For this review, take the finished solid that the model builds, in its own axes (mm). Give positions to 0.01 mm unless a question says otherwise; leave off trailing zeros. Write each loop counter-clockwise with the first axis right and the second up, starting at its lowest first coordinate (ties: lowest second). Pieces come first, ordered by that corner, then holes. Notation, with made-up numbers: (21, 44.25) -> (25, 44.25) arc R25 ccw to (25, 70.25) -> close; hole circle Ø6 at (49.25, -14.75). An arc over 180 degrees is marked (long way). Return JSON: item names as keys, results as strings.
Autodesk Inventor part; units mm, degrees
ref_plane "YZ Plane" through (0, 0, 0) normal (1, 0, 0) x (0, 1, 0)
ref_plane "XZ Plane" through (0, 0, 0) normal (0, 1, 0) x (-1, 0, 0)
ref_plane "XY Plane" through (0, 0, 0) normal (0, 0, 1) x (1, 0, 0)
sketch "Sketch1" plane through (0, 0, 0) normal (0, 1, 0) x (-1, 0, 0)
  circle A0 centre (0, 0) radius 27.5
  dimension "d0" = 55
extrude "Extrusion1" add sketch "Sketch1" along normal blind 6
sketch "Sketch2" plane through (0, 6, 0) normal (0, 1, 0) x (1, 0, 0)
  circle A0 centre (0, 0) radius 27.5
  point P0 (20, 0)
  point P1 (14.1421, 14.1421)
  point P2 (0, 20)
  point P3 (-14.1421, 14.1421)
  point P4 (-20, 0)
  point P5 (-14.1421, -14.1421)
  point P6 (0, -20)
  point P7 (14.1421, -14.1421)
  dimension "d3" = 20
  dimension "d6" = 360
hole "Hole1" at (20, 6, 0) at (14.1421, 6, -14.1421) at (0, 6, -20) at (-14.1421, 6, -14.1421) at (-20, 6, 0) at (-14.1421, 6, 14.1421) at (0, 6, 20) at (14.1421, 6, 14.1421) direction (0, -1, 0) diameter 6.6 depth 8 tip angle 118
properties part number "simple_plate"
1. To check wall thickness, follow probe 1 along X at (y, z) = (2.95, 11.5); probe 2 along Z at (x, y) = (-1, 2.85); probe 3 along X at (y, z) = (2.05, 12.5). State the ranges of each line that lie inside material, in increasing order.
Results found:
{"probe 1": "x = -24.98 to -16.12, -12.16 to 12.16, 16.12 to 24.98", "probe 2": "z = -27.48 to -23.14, -16.86 to 16.86, 23.14 to 27.48", "probe 3": "x = -24.49 to -17, -11.28 to 11.28, 17 to 24.49"}
2. The part is to be moulded in two halves that separate along Z. For faces 1 (the cylindrical face through (-12.9, 3, 17.2)), 2 (the cylindrical face through (1.26, 2.96, 23.05)), 3 (the cylindrical face through (5.961, 2.958, 26.846)), 4 (the flat face through (0, 0, 0)), say which applies: +Z half, -Z half, draft (parallel to the pull), parting line (faces both ways), or undercut.
Results found:
{"face 1": "undercut", "face 2": "undercut", "face 3": "parting line", "face 4": "draft"}
3. Add section C-C, the plane z = 1. State the section outline as (x, y) points.
Results found:
{"outline": "(-27.48, 0) -> (-23.14, 0) -> (-23.14, 6) -> (-27.48, 6) -> close; (-16.86, 0) -> (16.86, 0) -> (16.86, 6) -> (-16.86, 6) -> close; (23.14, 0) -> (27.48, 0) -> (27.48, 6) -> (23.14, 6) -> close"}
4. Add section B-B, the plane z = -20. State the section outline as (x, y) points, plus the area to 3 significant figures.
Results found:
{"outline": "(-18.87, 0) -> (-3.3, 0) -> (-3.3, 6) -> (-18.87, 6) -> close; (3.3, 0) -> (18.87, 0) -> (18.87, 6) -> (3.3, 6) -> close", "area": "187 mm²"}
5. Add section D-D, the plane x = 21.5. State the section outline as (y, z) points.
Results found:
{"outline": "(0, -17.15) -> (6, -17.15) -> (6, -2.94) -> (0, -2.94) -> close; (0, 2.94) -> (6, 2.94) -> (6, 17.15) -> (0, 17.15) -> close"}
6. Add section A-A, the plane x = 0. State the section outline as (y, z) points, plus the area to 3 significant figures.
Results found:
{"outline": "(0, -27.5) -> (6, -27.5) -> (6, -23.3) -> (0, -23.3) -> close; (0, -16.7) -> (6, -16.7) -> (6, 16.7) -> (0, 16.7) -> close; (0, 23.3) -> (6, 23.3) -> (6, 27.5) -> (0, 27.5) -> close", "area": "251 mm²"}
7. For pin 1 (3 mm diameter, centred on x = -19, y = 1.5, fed in from +Z); pin 2 (2 mm diameter, centred on x = -14.5, y = 4.5, fed in from +Z), all flat-tipped, find the tip position at first contact; note any pin that passes through.
Results found:
{"pin 1": "stops at z = 21.21", "pin 2": "stops at z = 23.96"}
